Verification items for the finished model (mm, model axes). Round coordinates to 2 decimals unless told otherwise and drop trailing zeros. Write each loop counter-clockwise with the first axis right and the second up, starting at its lowest first coordinate (ties: lowest second). Pieces come first, ordered by that corner, then holes. Notation, with made-up numbers: M 44,86.25 L 67,86.25 A21 cw 67,110.25 Z; hole C 38.25,72.25 d2. An arc over 180 degrees is marked long. Answer in a Markdown table with one row per item. Add a question column.
1. Material ranges on probe 1 along X at (y, z) = (-967.5, 4.25); probe 2 along X at (y, z) = (-987, 10); probe 3 along X at (y, z) = (-843, 11.75), recorded low to high.
2. Sectioned sample at A-A on y = -866. Record the cut outline in (x, z).
3. Sectioned sample at B-B on z = 9. Count the separate pieces of the cut face and the enclosed holes in it, plus the area to 3 significant figures.
4. Sectioned sample at D-D on x = 289. Record the cut outline in (y, z).
5. Go/stop test with flat-tipped pins: pin 1 Ø12 at (x, y) = (350.5, -959) entering from +Z; pin 2 Ø6 at (x, y) = (362.7, -996.5) entering from -Z; pin 3 Ø3 at (y, z) = (-944.5, 6) entering from +X; pin 4 Ø1 at (y, z) = (-843.5, 10.5) entering from +X. Record where each tip stops, or that it passes through.
6. Sectioned sample at C-C on y = -761. Record the cut outline in (x, z), plus the area to 3 significant figures.
```python
from build123d import *

# Parameters (mm, degrees)
BOSS_EXTRUDE1_DEPTH                              = 12.7
F_1_1_DIAMETER_HOLE1_D                           = 25.4
CBORE_FOR_1_4_SOCKET_HEAD_CAP_SCREW1_D           = 6.5278
CBORE_FOR_1_4_SOCKET_HEAD_CAP_SCREW1_CBORE_D     = 11.1125
CBORE_FOR_1_4_SOCKET_HEAD_CAP_SCREW1_CBORE_DEPTH = 7.112


with BuildPart() as part:
    # Sketch → Boss-Extrude1 (new body)
    with BuildSketch(Plane.XY):
        with BuildLine():
            Line((589.805840958, -702.903229895), (687.766672674, -819.648403026))
            ThreePointArc((687.766672674, -819.648403026), (0, -1069.975), (-687.766672674, -819.648403026))
            Line((-687.766672674, -819.648403026), (-589.805840958, -702.903229895))
            ThreePointArc((-589.805840958, -702.903229895), (0, -917.575), (589.805840958, -702.903229895))
        make_face()
    extrude(amount=BOSS_EXTRUDE1_DEPTH)

    # 1 (1) Diameter Hole1 (through all)
    with Locations(Plane.XY.offset(12.7)):
        with Locations((568.184817849, -811.452015073), (-418.64565008, -897.788493839), (418.64565008, -897.788493839), (-568.184817849, -811.452015073), (256.386146079, -956.846123522), (86.336478766, -986.83046793), (-86.336478766, -986.83046793), (-256.386146079, -956.846123522)):
            Hole(F_1_1_DIAMETER_HOLE1_D / 2)

    # CBORE for 1/4 Socket Head Cap Screw1 (through all)
    with Locations(Plane(origin=(11.711156934, 16.229076172, 12.7), x_dir=(-1, 0, 0), z_dir=(0, 0, 1))):
        with Locations((-350.984104056, 1012.726115884), (-324.922169134, 941.121538181), (-311.891201673, 905.319249329), (-337.953136595, 976.923827032), (335.313515542, 905.319249329), (348.344483002, 941.121538181), (361.375450463, 976.923827032), (374.406417924, 1012.726115884)):
            CounterBoreHole(CBORE_FOR_1_4_SOCKET_HEAD_CAP_SCREW1_D / 2, CBORE_FOR_1_4_SOCKET_HEAD_CAP_SCREW1_CBORE_D / 2, CBORE_FOR_1_4_SOCKET_HEAD_CAP_SCREW1_CBORE_DEPTH)


solid = part.part
```
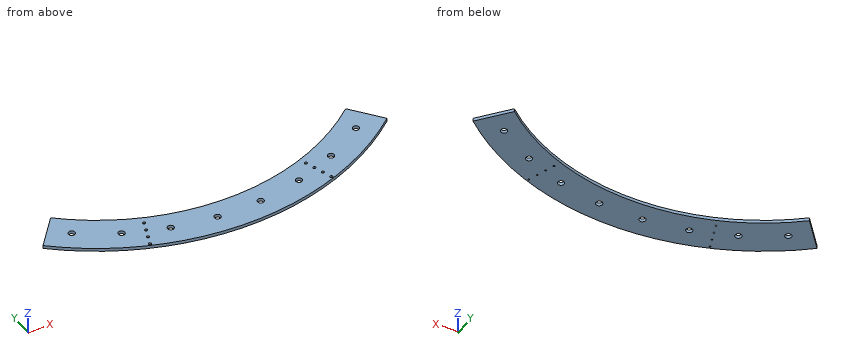
Geometry check:
| question | item | result |
|---|---|---|
| 1 | probe 1 | x = -456.94 to -263.3, -249.47 to 249.47, 263.3 to 456.94 |
| 1 | probe 2 | x = -413.13 to -99.04, -73.64 to 73.64, 99.04 to 413.13 |
| 1 | probe 3 | x = -658.94 to -362.35, 362.35 to 658.94 |
| 2 | outline | M -628.4,0 L -303.3,0 L -303.3,12.7 L -628.4,12.7 Z; M 303.3,0 L 628.4,0 L 628.4,12.7 L 303.3,12.7 Z |
| 3 | separate pieces | 1 |
| 3 | enclosed holes | 16 |
| 3 | area | 207,000 mm2 |
| 4 | outline | M -1030.21,0 L -870.87,0 L -870.87,12.7 L -1030.21,12.7 Z |
| 5 | pin 1 | stops at z = 12.7 |
| 5 | pin 2 | passes through |
| 5 | pin 3 | stops at x = 505.57 |
| 5 | pin 4 | stops at x = 658.94 |
| 6 | outline | M -638.55,0 L -512.66,0 L -512.66,12.7 L -638.55,12.7 Z; M 512.66,0 L 638.55,0 L 638.55,12.7 L 512.66,12.7 Z |
| 6 | area | 3,200 mm2 |
